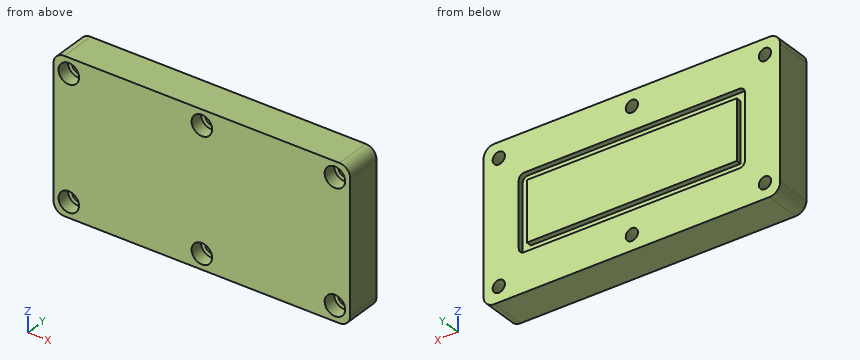
```python
from build123d import *

# Parameters (mm, degrees)
SKETCH1_W           = 104.775
SKETCH1_H           = 53.975
BOSS_EXTRUDE1_DEPTH = 12.7
SKETCH3_W           = 79.883
SKETCH3_H           = 26.797
SKETCH3_W_2         = 74.1045
SKETCH3_H_2         = 21.082
CUT_EXTRUDE1_DEPTH  = 1.905
FILLET1_R           = 1.905
SKETCH4_R           = 2.159
CUT_EXTRUDE2_DEPTH  = 61.283209209
SKETCH8_R           = 3.6195
CUT_EXTRUDE3_DEPTH  = 4.572
FILLET2_R           = 3.81


with BuildPart() as part:
    # Sketch1 → Boss-Extrude1 (new body)
    with BuildSketch(Plane(origin=(0, 0, 0), x_dir=(1, 0, 0), z_dir=(0, 1, 0))):
        Rectangle(SKETCH1_W, SKETCH1_H)
    extrude(amount=BOSS_EXTRUDE1_DEPTH)

    # Sketch3 → Cut-Extrude1 (cut)
    with BuildSketch(Plane(origin=(0, 12.7, 0), x_dir=(1, 0, 0), z_dir=(0, 1, 0))):
        Rectangle(SKETCH3_W, SKETCH3_H)
        Rectangle(SKETCH3_W_2, SKETCH3_H_2, mode=Mode.SUBTRACT)
    extrude(amount=-CUT_EXTRUDE1_DEPTH, mode=Mode.SUBTRACT)

    # Fillet1
    fillet1_edges = [part.edges().sort_by_distance(p)[0] for p in [
        (39.9415, 11.7475, -13.3985),
        (39.9415, 11.7475, 13.3985),
        (-39.9415, 11.7475, 13.3985),
        (-39.9415, 11.7475, -13.3985),
    ]]
    fillet(fillet1_edges, radius=FILLET1_R)

    # Sketch4 → Cut-Extrude2 (cut, through all)
    with BuildSketch(Plane.XZ):
        with Locations(Location((-46.99, 21.59, 0), (0, 0, 270))):
            Circle(SKETCH4_R)
        with Locations(Location((46.99, 21.59, 0), (0, 0, 270))):
            Circle(SKETCH4_R)
        with Locations(Location((-46.99, -21.59, 0), (0, 0, 270))):
            Circle(SKETCH4_R)
        with Locations(Location((46.99, -21.59, 0), (0, 0, 270))):
            Circle(SKETCH4_R)
        with Locations(Location((0, 21.59, 0), (0, 0, 270))):
            Circle(SKETCH4_R)
        with Locations(Location((0, -21.59, 0), (0, 0, 270))):
            Circle(SKETCH4_R)
    extrude(amount=-CUT_EXTRUDE2_DEPTH, mode=Mode.SUBTRACT)

    # Sketch8 → Cut-Extrude3 (cut)
    with BuildSketch(Plane.XZ):
        with Locations(Location((-46.99, 21.59, 0), (0, 0, 270))):
            Circle(SKETCH8_R)
        with Locations(Location((0, 21.59, 0), (0, 0, 270))):
            Circle(SKETCH8_R)
        with Locations(Location((46.99, 21.59, 0), (0, 0, 270))):
            Circle(SKETCH8_R)
        with Locations(Location((46.99, -21.59, 0), (0, 0, 270))):
            Circle(SKETCH8_R)
        with Locations(Location((0, -21.59, 0), (0, 0, 270))):
            Circle(SKETCH8_R)
        with Locations(Location((-46.99, -21.59, 0), (0, 0, 270))):
            Circle(SKETCH8_R)
    extrude(amount=-CUT_EXTRUDE3_DEPTH, mode=Mode.SUBTRACT)

    # Fillet2
    fillet2_edges = [part.edges().sort_by_distance(p)[0] for p in [
        (52.3875, 6.35, 26.9875),
        (-52.3875, 6.35, 26.9875),
        (-52.3875, 6.35, -26.9875),
        (52.3875, 6.35, -26.9875),
    ]]
    fillet(fillet2_edges, radius=FILLET2_R)


solid = part.part
```
Input: part model. Units: mm. Frame: model coordinates. Coordinates: 2 decimals unless noted, no trailing zeros. Loops run counter-clockwise (first coordinate to the right, second up) from the corner with the lowest first, then second, coordinate; pieces in that order, holes last. Notation, with made-up numbers: M 47.5,89 L 62.5,89 A17 cw 62.5,96 Z; hole C 52.5,40 d9. An arc over 180 degrees is marked long. One line per item, written item: value.
(1) Section D-D (x = 12). Output: boundary loops of the cut face in (y, z) (1 decimal).
Filled in:
outline: M 0,-27 L 12.7,-27 L 12.7,-13.4 L 10.8,-13.4 L 10.8,-10.5 L 12.7,-10.5 L 12.7,10.5 L 10.8,10.5 L 10.8,13.4 L 12.7,13.4 L 12.7,27 L 0,27 Z
(2) Section B-B (z = -21.59). Output: boundary loops of the cut face in (x, y), and give its area (3 significant figures).
Filled in:
outline: M -52.39,0 L -50.61,0 L -50.61,4.57 L -49.15,4.57 L -49.15,12.7 L -52.39,12.7 Z; M -44.83,4.57 L -43.37,4.57 L -43.37,0 L -3.62,0 L -3.62,4.57 L -2.16,4.57 L -2.16,12.7 L -44.83,12.7 Z; M 2.16,4.57 L 3.62,4.57 L 3.62,0 L 43.37,0 L 43.37,4.57 L 44.83,4.57 L 44.83,12.7 L 2.16,12.7 Z; M 49.15,4.57 L 50.61,4.57 L 50.61,0 L 52.39,0 L 52.39,12.7 L 49.15,12.7 Z
area: 1,130 mm^2
(3) Pin query (flat end, axial travel): pin 1 (5.5 mm diameter, centred on x = 0, z = -21.59, fed in from -Y). Return the tip coordinate at first contact, or that it passes through.
Filled in:
pin 1: y = 4.57
(4) Section C-C (y = 8.25). Output: boundary loops of the cut face in (x, z).
Filled in:
outline: M -52.39,-23.18 A3.81 ccw -48.58,-26.99 L 48.58,-26.99 A3.81 ccw 52.39,-23.18 L 52.39,23.18 A3.81 ccw 48.58,26.99 L -48.58,26.99 A3.81 ccw -52.39,23.18 Z; hole C -46.99,-21.59 d4.32; hole C -46.99,21.59 d4.32; hole C 0,-21.59 d4.32; hole C 0,21.59 d4.32; hole C 46.99,-21.59 d4.32; hole C 46.99,21.59 d4.32
(5) Line query: line 1 along Z through (x, y) = (23.5, 11.5); line 2 along X through (y, z) = (10.5, -21.59); line 3 along X through (y, z) = (1.4, 21.59). Output: solid intervals per line, ascending. Write a range as from..to.
Filled in:
line 1: -26.99..-13.4, -10.54..10.54, 13.4..26.99
line 2: -52.39..-49.15, -44.83..-2.16, 2.16..44.83, 49.15..52.39
line 3: -52.39..-50.61, -43.37..-3.62, 3.62..43.37, 50.61..52.39
(6) Section A-A (x = 46.99). Output: boundary loops of the cut face in (y, z).
Filled in:
outline: M 0,-26.99 L 12.7,-26.99 L 12.7,-23.75 L 4.57,-23.75 L 4.57,-25.21 L 0,-25.21 Z; M 0,-17.97 L 4.57,-17.97 L 4.57,-19.43 L 12.7,-19.43 L 12.7,19.43 L 4.57,19.43 L 4.57,17.97 L 0,17.97 Z; M 0,25.21 L 4.57,25.21 L 4.57,23.75 L 12.7,23.75 L 12.7,26.99 L 0,26.99 Z
